Autodesk Inventor part; units mm, degrees
ref_plane "YZ Plane" through (0, 0, 0) normal (1, 0, 0) x (0, 1, 0)
ref_plane "XZ Plane" through (0, 0, 0) normal (0, 1, 0) x (-1, 0, 0)
ref_plane "XY Plane" through (0, 0, 0) normal (0, 0, 1) x (1, 0, 0)
sketch "Sketch1" plane through (0, 0, 0) normal (0, 0, 1) x (1, 0, 0)
  line L0 (0, 0) -> (63.5, 0)
  line L1 (63.5, 0) -> (63.5, 31.75)
  line L2 (0, 31.75) -> (0, 0)
  line L3 (60.325, 31.75) -> (60.325, 3.175)
  line L4 (60.325, 3.175) -> (3.175, 3.175)
  line L5 (3.175, 3.175) -> (3.175, 31.75)
  line L6 (63.5, 31.75) -> (60.325, 31.75)
  line L7 (3.175, 31.75) -> (0, 31.75)
  dimension "d0" = 31.75
  dimension "d1" = 63.5
  dimension "d2" = 3.175
  dimension "d3" = 3.175
  dimension "d4" = 3.175
extrude "Extrusion1" add sketch "Sketch1" along normal blind 25.4
sketch "Sketch2" plane through (63.5, 0, 0) normal (1, 0, 0) x (0, 0, -1)
  line L0 (-25.4, 31.75) -> (-25.4, 0)
  line L1 (0, 0) -> (-25.4, 0)
  line L2 (0, 0) -> (0, 31.75)
  line L3 (0, 31.75) -> (-25.4, 31.75)
  arc A0 (-4.9503, 25.5287) -> (-20.4497, 25.5287) centre (-12.7, 23.8125) ccw
  line L4 (-25.4, 3.175) -> (-20.4497, 25.5287)
  line L5 (0, 3.175) -> (-4.9503, 25.5287)
  circle A1 centre (-12.7, 23.8125) radius 4.7625
  dimension "d7" = 15.875
  dimension "d8" = 3.175
  dimension "d9" = 9.525
  dimension "d10" = 12.7
extrude "Extrusion2" cut sketch "Sketch2" against normal through all contours L3 A0 L4 L0 | L3 L2 L5 A0 | A1
equation "\"d3\" = d2"
equation "\"d4\" = d3"
properties part number "manipulator apendage pivot"
Check sheet for the modelled part. Datum: model origin and axes. Units: mm. A direction names the side the tool comes from. Coordinates: 2 decimals unless noted, no trailing zeros. Write each loop counter-clockwise with the first axis right and the second up, starting at its lowest first coordinate (ties: lowest second). Pieces come first, ordered by that corner, then holes.
Item 1: Mould release check, pull along X, two halves, no side actions. Record for faces 1 (the face through (1.61, 14.2, 22.96)), 2 (the face through (0, 13, 13)), 3 (the face through (32, 3.175, 13)): released by +X, released by -X, zero draft, split by the parting line, or undercut.
Numbers:
face 1: zero draft
face 2: released by -X
face 3: undercut
Item 2: Access from +Z, -Z, +X, -X, +Y, -Y to the whole of each face (thin tool, end or side, straight path). Record for faces 4 (the face through (3.175, 14, 13)), 5 (the face through (31, 2, 0)).
Numbers:
face 4: +Z, -Z, +Y
face 5: -Z, +X, -X, +Y, -Y
Item 3: Cross-section at D-D on x = 58.5. Record the boundary of the cut face in (y, z) (3 decimals), then the cut area to 3 significant figures.
Numbers:
outline: (0, 0) - (3.175, 0) - (3.175, 25.4) - (0, 25.4) - close
area: 80.6 mm2
Item 4: Depth check by flat-ended pin: pin 1 Ø6 at (x, z) = (33.5, 22) entering from +Y (3 decimals). Enter the tip coordinate at first touch or a pass-through.
Numbers:
pin 1: stops at y = 3.175
Item 5: Scan lines: probe 1 along Y at (x, z) = (0.9, 12.7) (3 decimals); probe 2 along X at (y, z) = (23.5, 19.75) (3 decimals); probe 3 along Y at (x, z) = (56.5, 19.5) (3 decimals). Record each from-to range of solid material in increasing order.
Numbers:
probe 1: y = 0 to 19.05, 28.575 to 31.75
probe 2: x = 0 to 3.175, 60.325 to 63.5
probe 3: y = 0 to 3.175
Item 6: Cross-section at A-A on z = 12.7. Record the boundary of the cut face in (x, y) (3 decimals), then the cut area to 3 significant figures.
Numbers:
outline: (0, 0) - (63.5, 0) - (63.5, 19.05) - (60.325, 19.05) - (60.325, 3.175) - (3.175, 3.175) - (3.175, 19.05) - (0, 19.05) - close; (0, 28.575) - (3.175, 28.575) - (3.175, 31.75) - (0, 31.75) - close; (60.325, 28.575) - (63.5, 28.575) - (63.5, 31.75) - (60.325, 31.75) - close
area: 323 mm2
Item 7: Cross-section at C-C on y = 7.5. Record the boundary of the cut face in (x, z) (3 decimals).
Numbers:
outline: (0, 0.958) - (3.175, 0.958) - (3.175, 24.442) - (0, 24.442) - close; (60.325, 0.958) - (63.5, 0.958) - (63.5, 24.442) - (60.325, 24.442) - close
Item 8: Cross-section at B-B on y = 20. Record the boundary of the cut face in (x, z) (3 decimals).
Numbers:
outline: (0, 3.726) - (3.175, 3.726) - (3.175, 9.846) - (0, 9.846) - close; (0, 15.554) - (3.175, 15.554) - (3.175, 21.674) - (0, 21.674) - close; (60.325, 3.726) - (63.5, 3.726) - (63.5, 9.846) - (60.325, 9.846) - close; (60.325, 15.554) - (63.5, 15.554) - (63.5, 21.674) - (60.325, 21.674) - close
